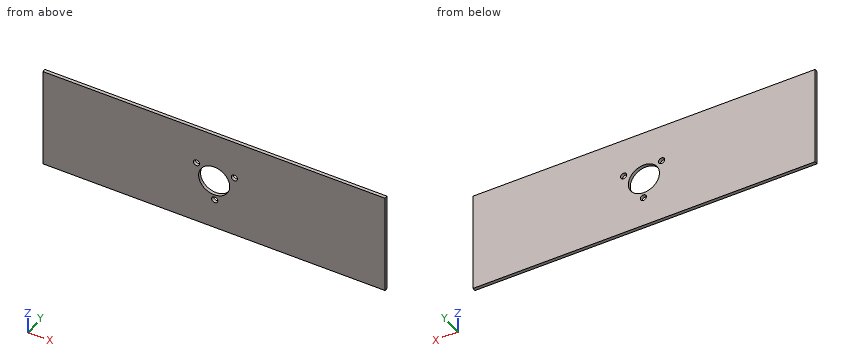
from build123d import *

# Parameters (mm, degrees)
SKETCH1_W             = 165
SKETCH1_H             = 50
BOSS_EXTRUDE1_DEPTH   = 1.6
F_5_0MM_DOWEL_HOLE1_D = 15
F_3_0MM_DOWEL_HOLE1_D = 3
F_3_0MM_DOWEL_HOLE2_D = 3
F_3_0MM_DOWEL_HOLE3_D = 3


with BuildPart() as part:
    # Sketch1 → Boss-Extrude1 (new body)
    with BuildSketch(Plane(origin=(0, 0, 0), x_dir=(1, 0, 0), z_dir=(0, 1, 0))):
        with Locations((-9.486062718, 16.824912892)):
            Rectangle(SKETCH1_W, SKETCH1_H)
    extrude(amount=BOSS_EXTRUDE1_DEPTH)

    # Ø5.0mm Dowel Hole1 (through all)
    with Locations(Plane(origin=(0, 1.6, 0), x_dir=(1, 0, 0), z_dir=(0, 1, 0))):
        with Locations((-9.417861972, 16.694999661)):
            Hole(F_5_0MM_DOWEL_HOLE1_D / 2)

    # Ø3.0mm Dowel Hole1 (through all)
    with Locations(Plane(origin=(0, 1.6, 0), x_dir=(1, 0, 0), z_dir=(0, 1, 0))):
        with Locations((-9.173425023, 26.839133027)):
            Hole(F_3_0MM_DOWEL_HOLE1_D / 2)

    # Ø3.0mm Dowel Hole2 (through all)
    with Locations(Plane(origin=(0, 1.6, 0), x_dir=(1, 0, 0), z_dir=(0, 1, 0))):
        with Locations((0.359615971, 11.072949843)):
            Hole(F_3_0MM_DOWEL_HOLE2_D / 2)

    # Ø3.0mm Dowel Hole3 (through all)
    with Locations(Plane(origin=(0, 1.6, 0), x_dir=(1, 0, 0), z_dir=(0, 1, 0))):
        with Locations((-17.973155173, 10.461857472)):
            Hole(F_3_0MM_DOWEL_HOLE3_D / 2)


solid = part.part
Geometry: final body of the model. Coordinates: model frame, mm. Round coordinates to 2 decimals unless told otherwise and drop trailing zeros. Order: outer loops, then holes, each group sorted by start corner. A loop starts at its lowest first (then second) coordinate and runs counter-clockwise, first axis right, second up. Notation, with made-up numbers: (6.25, 65.5) - (38.25, 65.5) arc R8 ccw to (38.25, 69.5) - close; hole circle Ø10 at (-33.5, 78.25). An arc over 180 degrees is marked (long way). Write each question's results on one line, items separated by ' | '.
Item 1: Section A-A, the plane x = -6. Return the cut outline in (y, z).
Completed:
outline: (0, -41.82) - (1.6, -41.82) - (1.6, -23.37) - (0, -23.37) - close; (0, -10.02) - (1.6, -10.02) - (1.6, 8.18) - (0, 8.18) - close
Item 2: Material intervals for line 1 along Z through (x, y) = (-18, 0.35); line 2 along X through (y, z) = (1.15, -11.5); line 3 along Z through (x, y) = (-14.5, 1.3), sorted ascending. Write a range as [from, to].
Completed:
line 1: [-41.82, -11.96], [-8.96, 8.18] | line 2: [-91.99, -19.06], [-16.89, -14.83], [-4.01, -1.08], [1.8, 73.01] | line 3: [-41.82, -22.21], [-11.18, 8.18]
Item 3: Section B-B, the plane z = -15. Return the cut outline in (x, y), and give its area (3 significant figures).
Completed:
outline: (-91.99, 0) - (-16.72, 0) - (-16.72, 1.6) - (-91.99, 1.6) - close; (-2.11, 0) - (73.01, 0) - (73.01, 1.6) - (-2.11, 1.6) - close | area: 241 mm^2
Item 4: Section C-C, the plane y = 0.65. Return the cut outline in (x, z) (3 decimals).
Completed:
outline: (-91.986, -41.825) - (73.014, -41.825) - (73.014, 8.175) - (-91.986, 8.175) - close; hole circle Ø3 at (-17.973, -10.462); hole circle Ø15 at (-9.418, -16.695); hole circle Ø3 at (-9.173, -26.839); hole circle Ø3 at (0.36, -11.073)
